```python
from build123d import *

# Parameters (mm, degrees)
SKETCH1_W                    = 31.75
SKETCH1_H                    = 63.5
SKETCH1_W_2                  = 25.4
SKETCH1_H_2                  = 57.15
BOSS_EXTRUDE1_DEPTH          = 76.2
CUT_EXTRUDE1_REACH           = 103.105
SKETCH3_R                    = 9.525
CUT_EXTRUDE2_DEPTH           = 3.175
F_10_0_1935_DIAMETER_HOLE1_D = 4.9149


with BuildPart() as part:
    # Sketch1 → Boss-Extrude1 (new body)
    with BuildSketch(Plane.XY):
        with Locations((3.710272719, -29.23968021)):
            Rectangle(SKETCH1_W, SKETCH1_H)
        with Locations((3.710272719, -29.23968021)):
            Rectangle(SKETCH1_W_2, SKETCH1_H_2, mode=Mode.SUBTRACT)
    extrude(amount=BOSS_EXTRUDE1_DEPTH)

    # Cut-Extrude1: up to this face of the body (flat: up to its plane)
    cut_extrude1_end = Plane(part.part.faces().sort_by_distance((3.710272719, -60.98968021, 38.1))[0])
    # Sketch2 → Cut-Extrude1 (cut, up to the picked face)
    with BuildSketch(Plane(origin=(0, 2.51031979, 0), x_dir=(1, 0, 0), z_dir=(0, 1, 0)), mode=Mode.PRIVATE) as cut_extrude1_sk1:
        Polygon((-12.164727281, -76.2), (13.235272719, -76.2), (-12.164727281, -44.45), align=None)
    cut_extrude1_tool1 = split(extrude(cut_extrude1_sk1.sketch, amount=-CUT_EXTRUDE1_REACH, mode=Mode.PRIVATE), bisect_by=cut_extrude1_end, keep=Keep.BOTH, mode=Mode.PRIVATE)
    add(cut_extrude1_tool1.solids().sort_by(Axis((-3.698061, 2.51032, 65.616667), (0, -1, 0)))[0], mode=Mode.SUBTRACT)

    # Sketch3 → Cut-Extrude2 (cut)
    with BuildSketch(Plane.ZY.offset(-16.410272719)):
        with Locations(Location((60.325, -29.23968021, 0), (0, 0, 270))):
            Circle(SKETCH3_R)
    extrude(amount=-CUT_EXTRUDE2_DEPTH, mode=Mode.SUBTRACT)

    # #10 (0.1935) Diameter Hole1 (through all)
    with Locations(Plane(origin=(16.410272719, -48.28968021, 60.325), x_dir=(0, -1, 0), z_dir=(-1, 0, 0))):
        with Locations((0, 0), (-38.1, 0)):
            Hole(F_10_0_1935_DIAMETER_HOLE1_D / 2)


solid = part.part
```
For this review, take the finished solid that the model builds, in its own axes (mm). A direction names the side the tool comes from. Round coordinates to 2 decimals unless told otherwise and drop trailing zeros. Write each loop counter-clockwise with the first axis right and the second up, starting at its lowest first coordinate (ties: lowest second). Pieces come first, ordered by that corner, then holes. Notation, with made-up numbers: (48.5, -14.75) -> (64.5, -14.75) arc R9 cw to (64.5, -7.75) -> close; hole circle Ø1 at (24, 56). An arc over 180 degrees is marked (long way). Use one line per item in the form item = value.
Q1. Consider section C-C (y = -1.5). State the section outline as (x, z) points, then the cut area to 3 significant figures.
Resolved:
outline = (-12.16, 0) -> (-8.99, 0) -> (-8.99, 48.42) -> (-12.16, 44.45) -> close; (16.41, 0) -> (19.59, 0) -> (19.59, 76.2) -> (16.41, 76.2) -> close
area = 389 mm²
Q2. Clearance check with flat-ended pins moving along their axes: pin 1 Ø8 at (y, z) = (-12, 63.5) entering from -X; pin 2 Ø25 at (y, z) = (-29.24, 60.32) entering from -X; pin 3 Ø3 at (y, z) = (-10.19, 60.32) entering from +X; pin 4 Ø12 at (y, z) = (-14, 53) entering from -X. State where each tip first meets the part, or that it passes through.
Resolved:
pin_1 = 16.41
pin_2 = -9.47
pin_3 = through
pin_4 = -10.12
Q3. Machinability: for faces 1 (the flat face through (16.41, -30, 38)), 2 (the flat face through (-12.165, -30, 22)), which of the approach directions +Z, -Z, +X, -X, +Y, -Y give a long, thin tool a straight path to every point of the face, cutting with its end or side? Answer none if there is none.
Resolved:
face_1 = +Z, -Z
face_2 = +Z, -Z, -X, +Y, -Y
Q4. Consider section B-B (z = 28.5). State the section outline as (x, y) points, then the cut area to 3 significant figures.
Resolved:
outline = (-12.16, -60.99) -> (19.59, -60.99) -> (19.59, 2.51) -> (-12.16, 2.51) -> close; hole (-8.99, -57.81) -> (16.41, -57.81) -> (16.41, -0.66) -> (-8.99, -0.66) -> close
area = 565 mm²
Q5. The part is to be moulded in two halves that separate along Z. For faces 3 (the flat face through (3, -60.99, 29)), 4 (the flat face through (-9.754, -29.092, 47.464)), 5 (the cylindrical face through (18.02, -48.822, 57.926)), 6 (the flat face through (-9.3, -26.7, 0)), say which applies: released by +Z, released by -Z, zero draft, split by the parting line, or undercut.
Resolved:
face_3 = zero draft
face_4 = released by +Z
face_5 = undercut
face_6 = released by -Z
Q6. Consider section A-A (x = 15.5). State the section outline as (y, z) points, then the cut area to 3 significant figures.
Resolved:
outline = (-60.99, 0) -> (-57.81, 0) -> (-57.81, 76.2) -> (-60.99, 76.2) -> close; (-0.66, 0) -> (2.51, 0) -> (2.51, 76.2) -> (-0.66, 76.2) -> close
area = 484 mm²
Q7. To check wall thickness, follow probe 1 along X at (y, z) = (-53.5, 4); probe 2 along Y at (x, z) = (-5.5, 13); probe 3 along X at (y, z) = (-13, 54). State the ranges of each line that lie inside material, in increasing order. Write a range as from..to.
Resolved:
probe_1 = -12.16..-8.99, 16.41..19.59
probe_2 = -60.99..-57.81, -0.66..2.51
probe_3 = 16.41..19.59
Q8. Consider section D-D (y = -25). State the section outline as (x, z) points.
Resolved:
outline = (-12.16, 0) -> (-8.99, 0) -> (-8.99, 48.42) -> (-12.16, 44.45) -> close; (16.41, 0) -> (19.59, 0) -> (19.59, 51.8) -> (16.41, 51.8) -> close; (16.41, 68.85) -> (19.59, 68.85) -> (19.59, 76.2) -> (16.41, 76.2) -> close
